```python
from build123d import *

# Parameters (mm, degrees)
SKETCH1_W           = 75
SKETCH1_H           = 75
SKETCH1_R           = 1.5
BOSS_EXTRUDE1_DEPTH = 10
FILLET1_R           = 5
FILLET2_R           = 15


with BuildPart() as part:
    # Sketch1 → Boss-Extrude1 (new body)
    with BuildSketch(Plane(origin=(0, 0, 0), x_dir=(1, 0, 0), z_dir=(0, 1, 0))):
        Rectangle(SKETCH1_W, SKETCH1_H)
        with Locations(Location((24.748737342, 24.748737342, 0), (0, 0, 270))):
            Circle(SKETCH1_R, mode=Mode.SUBTRACT)
        with Locations(Location((-24.748737342, -24.748737342, 0), (0, 0, 270))):
            Circle(SKETCH1_R, mode=Mode.SUBTRACT)
        with Locations(Location((-9.058666579, -33.80740392, 0), (0, 0, 270))):
            Circle(SKETCH1_R, mode=Mode.SUBTRACT)
        with Locations(Location((-33.80740392, -9.058666579, 0), (0, 0, 270))):
            Circle(SKETCH1_R, mode=Mode.SUBTRACT)
        with Locations(Location((9.058666579, -33.80740392, 0), (0, 0, 270))):
            Circle(SKETCH1_R, mode=Mode.SUBTRACT)
        with Locations(Location((24.748737342, -24.748737342, 0), (0, 0, 270))):
            Circle(SKETCH1_R, mode=Mode.SUBTRACT)
        with Locations(Location((33.80740392, -9.058666579, 0), (0, 0, 270))):
            Circle(SKETCH1_R, mode=Mode.SUBTRACT)
        with Locations(Location((-33.80740392, 9.058666579, 0), (0, 0, 270))):
            Circle(SKETCH1_R, mode=Mode.SUBTRACT)
        with Locations(Location((-24.748737342, 24.748737342, 0), (0, 0, 270))):
            Circle(SKETCH1_R, mode=Mode.SUBTRACT)
        with Locations(Location((-9.058666579, 33.80740392, 0), (0, 0, 270))):
            Circle(SKETCH1_R, mode=Mode.SUBTRACT)
        with BuildLine():
            ThreePointArc((28.282562779, 10.004830964), (30, 0), (28.282562779, -10.004830964))
            ThreePointArc((28.282562779, -10.004830964), (30.743901834, -17.75), (22.805719165, -19.491002369))
            ThreePointArc((22.805719165, -19.491002369), (15, -25.980762114), (5.476843614, -29.495833333))
            ThreePointArc((5.476843614, -29.495833333), (0, -35.5), (-5.476843614, -29.495833333))
            ThreePointArc((-5.476843614, -29.495833333), (-15, -25.980762114), (-22.805719165, -19.491002369))
            ThreePointArc((-22.805719165, -19.491002369), (-30.743901834, -17.75), (-28.282562779, -10.004830964))
            ThreePointArc((-28.282562779, -10.004830964), (-30, 0), (-28.282562779, 10.004830964))
            ThreePointArc((-28.282562779, 10.004830964), (-30.743901834, 17.75), (-22.805719165, 19.491002369))
            ThreePointArc((-22.805719165, 19.491002369), (-15, 25.980762114), (-5.476843614, 29.495833333))
            ThreePointArc((-5.476843614, 29.495833333), (0, 35.5), (5.476843614, 29.495833333))
            ThreePointArc((5.476843614, 29.495833333), (15, 25.980762114), (22.805719165, 19.491002369))
            ThreePointArc((22.805719165, 19.491002369), (30.743901834, 17.75), (28.282562779, 10.004830964))
        make_face(mode=Mode.SUBTRACT)
        with Locations(Location((33.80740392, 9.058666579, 0), (0, 0, 270))):
            Circle(SKETCH1_R, mode=Mode.SUBTRACT)
        with Locations(Location((9.058666579, 33.80740392, 0), (0, 0, 270))):
            Circle(SKETCH1_R, mode=Mode.SUBTRACT)
    extrude(amount=BOSS_EXTRUDE1_DEPTH)

    # Fillet1
    fillet1_edges = [part.edges().sort_by_distance(p)[0] for p in [
        (-28.282562779, 5, -10.004830964),
        (-28.282562779, 5, 10.004830964),
        (-22.805719165, 5, 19.491002369),
        (-5.476843614, 5, 29.495833333),
        (5.476843614, 5, 29.495833333),
        (22.805719165, 5, 19.491002369),
        (28.282562779, 5, 10.004830964),
        (28.282562779, 5, -10.004830964),
        (22.805719165, 5, -19.491002369),
        (5.476843614, 5, -29.495833333),
        (-5.476843614, 5, -29.495833333),
        (-22.805719165, 5, -19.491002369),
    ]]
    fillet(fillet1_edges, radius=FILLET1_R)

    # Fillet2
    fillet2_edges = [part.edges().sort_by_distance(p)[0] for p in [
        (-37.5, 5, -37.5),
        (37.5, 5, -37.5),
        (37.5, 5, 37.5),
        (-37.5, 5, 37.5),
    ]]
    fillet(fillet2_edges, radius=FILLET2_R)


solid = part.part
```
CAD build for the part. Positions are in the model's coordinates, mm. A direction names the side the tool comes from. Coordinates: 2 decimals unless noted, no trailing zeros. Order: outer loops, then holes, each group sorted by start corner. A loop starts at its lowest first (then second) coordinate and runs counter-clockwise, first axis right, second up. Notation, with made-up numbers: (85.25, 54) -> (123.25, 54) arc R32 cw to (123.25, 81) -> close; hole circle Ø1 at (4, 75). An arc over 180 degrees is marked (long way). Use one line per item in the form item = value. Start each with the question number.
1) Band-saw the part on C-C on y = 9. State how many separate pieces and enclosed holes the cut face has, then the cut area to 3 significant figures.
2) Tool access for faces 1 (the cylindrical face through (32.99, 5.07, -33.22)), 2 (the cylindrical face through (14.913, 4.93, -26.031)): list every direction of +Z, -Z, +X, -X, +Y, -Y with a clear straight run to the whole face (end or side of a thin tool).
3) Drop a flat-ended pin along its axis: pin 1 (2.5 mm diameter, centred on x = 33.81, z = 9.06, fed in from -Y). Give the stop position or say it passes through.
4) Pull direction Z, two halves, no side cores. Call faces 3 (the flat face through (-20, 10, 25)), 4 (the cylindrical face through (32.99, 5.07, 33.22)), 5 (the cylindrical face through (30.696, 4.93, -17.831)): +Z half, -Z half, draft (parallel to the pull), parting line (faces both ways), or undercut.
5) Band-saw the part on B-B on x = -11.5. Give the cut face in (y, z).
6) Band-saw the part on A-A on z = 15. Give the cut face in (x, y).
7) Drill centre lines: L1, parallel to Z at x = -32.5, y = 6; L2, parallel to X at y = 9.25, z = 25; L3, parallel to Z at x = -25.5, y = 3.25. Where is each one in solid material? Low to high. Write a range as [from, to].
Entries:
q1.separate_pieces = 1
q1.enclosed_holes = 13
q1.area = 2,210 mm2
q2.face_1 = -Z, +X, +Y, -Y
q2.face_2 = +Y, -Y
q3.pin_1 = through
q4.face_3 = draft
q4.face_4 = +Z half
q4.face_5 = undercut
q5.outline = (0, -37.5) -> (10, -37.5) -> (10, -27.71) -> (0, -27.71) -> close; (0, 27.71) -> (10, 27.71) -> (10, 37.5) -> (0, 37.5) -> close
q6.outline = (-37.5, 0) -> (-31.48, 0) -> (-31.48, 10) -> (-37.5, 10) -> close; (31.48, 0) -> (37.5, 0) -> (37.5, 10) -> (31.48, 10) -> close
q7.L1 = [-33.68, -9.79], [-8.32, 8.32], [9.79, 33.68]
q7.L2 = [-37.29, -26.23], [-23.27, -16.58], [16.58, 23.27], [26.23, 37.29]
q7.L3 = [-37.2, -26.05], [-23.45, -20.48], [20.48, 23.45], [26.05, 37.2]
